Verification items for the finished model (mm, model axes). A direction names the side the tool comes from. Round coordinates to 2 decimals unless told otherwise and drop trailing zeros. Order: outer loops, then holes, each group sorted by start corner. A loop starts at its lowest first (then second) coordinate and runs counter-clockwise, first axis right, second up. Notation, with made-up numbers: (83.5, -8) -> (137.5, -8) arc R25 cw to (137.5, 26) -> close; hole circle Ø8 at (27.25, -36.75). An arc over 180 degrees is marked (long way). Put each result on its own line as item: value.
Autodesk Inventor part; units mm, degrees
ref_plane "YZ Plane" through (0, 0, 0) normal (1, 0, 0) x (0, 1, 0)
ref_plane "XZ Plane" through (0, 0, 0) normal (0, 1, 0) x (-1, 0, 0)
ref_plane "XY Plane" through (0, 0, 0) normal (0, 0, 1) x (1, 0, 0)
sketch "Sketch1" plane through (0, 0, 0) normal (0, 0, 1) x (1, 0, 0)
  point P0 (0, 0)
sketch "Sketch2" plane through (0, 0, 0) normal (0, 0, 1) x (1, 0, 0)
  line L0 (0, 0) -> (215.9, 0)
  line L1 (215.9, 0) -> (215.9, 50.8)
  line L2 (215.9, 50.8) -> (0, 50.8)
  line L3 (0, 50.8) -> (0, 0)
  dimension "d0" = 215.9
  dimension "d1" = 50.8
extrude "Extrusion1" add sketch "Sketch2" along normal blind 9.525
sketch "Sketch3" plane through (0, 0, 9.525) normal (0, 0, 1) x (1, 0, 0)
  line L0 (215.9, 0) -> (215.9, 50.8)
  line L1 (215.9, 0) -> (215.9, 30.48)
  line L2 (0, 0) -> (0, 30.48)
  line L3 (0, 50.8) -> (0, 0)
  line L4 (0, 30.48) -> (215.9, 30.48)
  line L5 (215.9, 0) -> (203.2, 0)
  line L6 (0, 0) -> (215.9, 0)
  line L7 (203.2, 0) -> (203.2, 50.8)
  line L8 (215.9, 50.8) -> (0, 50.8)
  line L9 (203.2, 0) -> (177.8, 0)
  line L10 (177.8, 0) -> (152.4, 0)
  line L11 (177.8, 0) -> (137.16, 0)
  line L12 (177.8, 0) -> (177.8, 9.525)
  line L13 (177.8, 9.525) -> (137.16, 9.525)
  line L14 (137.16, 9.525) -> (177.8, 9.525)
  line L15 (177.8, 9.525) -> (177.8, 30.48)
  line L16 (177.8, 30.48) -> (137.16, 30.48)
  line L17 (137.16, 30.48) -> (137.16, 9.525)
  line L18 (137.16, 9.525) -> (177.36, 9.525)
  line L19 (177.36, 9.525) -> (177.36, 29.525)
  line L20 (177.36, 29.525) -> (137.16, 29.525)
  line L21 (137.16, 29.525) -> (137.16, 9.525)
  point P0 (177.36, 9.525)
  dimension "d4" = 30.48
  dimension "d5" = 30.48
  dimension "d6" = 12.7
  dimension "d7" = 25.4
  dimension "d8" = 25.4
  dimension "d9" = 40.64
  dimension "d10" = 9.525
  dimension "d11" = 40.64
  dimension "d12" = 40.2
  dimension "d13" = 20
extrude "Extrusion2" cut sketch "Sketch3" against normal blind 25.4 contours L13 L17 L20 L19
sketch "Sketch4" plane through (0, 0, 9.525) normal (0, 0, 1) x (1, 0, 0)
  line L0 (0, 0) -> (0, 30.48)
  line L1 (0, 50.8) -> (0, 0)
  line L2 (137.16, 29.525) -> (177.36, 29.525)
  line L3 (0, 30.48) -> (137.16, 29.525)
  line L4 (215.9, 50.8) -> (0, 50.8)
  line L5 (0, 30.48) -> (111.76, 30.48)
  line L6 (111.76, 30.48) -> (111.76, 50.8)
  line L7 (111.76, 50.8) -> (0, 50.8)
  line L8 (0, 50.8) -> (0, 30.48)
  arc A0 (111.76, 40.64) -> (109.4345, 29.525) centre (137.16, 29.525) ccw
  point P0 (109.451, 30.48)
  dimension "d16" = 30.48
extrude "Extrusion3" cut sketch "Sketch4" against normal blind 25.4 contours L4 L6 A0 L5 L1
sketch "Sketch5" plane through (0, 0, 9.525) normal (0, 0, 1) x (1, 0, 0)
  line L0 (137.16, 9.525) -> (177.36, 9.525)
  line L1 (137.16, 9.525) -> (132.36, 9.525)
  line L2 (132.36, 9.525) -> (132.36, 13.9192)
  circle A0 centre (132.36, 13.9192) radius 2.25
  line L3 (132.36, 13.9192) -> (132.36, 23.8192)
  circle A1 centre (132.36, 23.8192) radius 2.2479
  line L4 (177.36, 9.525) -> (182.1606, 9.525)
  line L5 (182.1606, 9.525) -> (182.1606, 13.9192)
  circle A2 centre (182.1606, 13.9192) radius 2.2479
  line L6 (182.1606, 13.9192) -> (182.1606, 23.8252)
  circle A3 centre (182.1606, 23.8252) radius 2.2479
  point P0 (0, 0)
  dimension "d19" = 4.8
  dimension "d20" = 4.3942
  dimension "d21" = 4.5
  dimension "d22" = 9.9
  dimension "d23" = 4.4958
  dimension "d24" = 4.8006
  dimension "d25" = 4.3942
  dimension "d26" = 4.4958
  dimension "d27" = 9.906
  dimension "d28" = 4.4958
extrude "Extrusion4" cut sketch "Sketch5" against normal blind 25.4
sketch "Sketch7" plane through (0, 0, 9.525) normal (0, 0, 1) x (1, 0, 0)
  line L0 (177.36, 29.525) -> (177.36, 9.525)
  line L1 (177.36, 9.525) -> (215.9, 9.525)
  line L2 (215.9, 0) -> (215.9, 50.8)
  circle A0 centre (182.1606, 13.9192) radius 2.2479
  line L3 (184.4085, 13.9192) -> (215.9, 13.9192)
  line L4 (175.586, 50.8) -> (175.586, 0)
  line L5 (0, 0) -> (215.9, 0)
  line L6 (141.0803, 19.525) -> (205.5055, 19.525)
  circle A1 centre (175.586, 19.525) radius 2.2479
  dimension "d33" = 4.4958
extrude "Extrusion6" cut sketch "Sketch7" against normal blind 25.4 contours A1 L6 L0 | L0 L6 L4 A1 | L6 A1 L0 | L0 A1 L4 L6 | L4 L6 A1 | L4 A1 L6
sketch "Sketch8" plane through (0, 0, 9.525) normal (0, 0, 1) x (1, 0, 0)
  point P0 (0, 0)
sketch "Sketch9" plane through (0, 0, 9.525) normal (0, 0, 1) x (1, 0, 0)
  point P0 (0, 0)
sketch "Sketch10" plane through (0, 0, 9.525) normal (0, 0, 1) x (1, 0, 0)
  point P0 (0, 0)
fillet "Fillet1" radius 3.175 4 edges at (137.16, 9.525, 4.7625) (137.16, 29.525, 4.7625) (177.36, 29.525, 4.7625) (177.36, 9.525, 4.7625)
fillet "Fillet2" radius 3.175 3 edges at (111.76, 50.8, 4.7625) (111.76, 40.64, 4.7625) (109.451, 30.48, 4.7625)
fillet "Fillet3" radius 15.24 4 edges at (0, 30.48, 4.7625) (0, 0, 4.7625) (215.9, 50.8, 4.7625) (215.9, 0, 4.7625)
sketch "Sketch11" plane through (0, 0, 9.525) normal (0, 0, 1) x (1, 0, 0)
  line L0 (106.5367, 30.48) -> (15.24, 30.48)
  line L1 (15.24, 0) -> (200.66, 0)
  line L2 (15.24, 30.48) -> (15.24, 0)
  line L3 (15.24, 0) -> (15.24, 15.24)
  line L4 (15.24, 15.24) -> (30.48, 15.24)
  line L5 (30.48, 15.24) -> (0, 15.24)
  arc A0 (15.24, 30.48) -> (15.24, 0) centre (15.24, 15.24) ccw
  circle A1 centre (15.24, 15.24) radius 3.81
  circle A2 centre (25.019, 15.24) radius 1.3589
  circle A3 centre (15.24, 25.019) radius 1.3589
  circle A4 centre (5.461, 15.24) radius 1.3589
  circle A5 centre (15.24, 5.461) radius 1.3589
  point P0 (0, 0)
  dimension "d39" = 15.24
  dimension "d40" = 7.62
  dimension "d41" = 2.7178
  dimension "d42" = 2.7178
  dimension "d43" = 2.7178
  dimension "d44" = 2.7178
extrude "Extrusion7" cut sketch "Sketch11" against normal blind 25.4 contours A2 L4 | L4 A2 | A3 L2 | L2 A3 | A4 L5 | L5 A4 | A1 L4 L2 | L2 L5 A1 | A5 L2 | L2 A5 | L4 A1 L2 | L2 A1 L5
sketch "Sketch12" plane through (0, 0, 9.525) normal (0, 0, 1) x (1, 0, 0)
  circle A0 centre (5.461, 15.24) radius 1.3589
  circle A1 centre (5.461, 15.24) radius 2.2479
  circle A2 centre (15.24, 5.461) radius 1.3589
  circle A3 centre (15.24, 5.461) radius 2.2479
  circle A4 centre (25.019, 15.24) radius 1.3589
  circle A5 centre (25.019, 15.24) radius 2.2479
  circle A6 centre (15.24, 25.019) radius 1.3589
  circle A7 centre (15.24, 25.019) radius 2.2479
  circle A8 centre (15.24, 25.019) radius 2.54
  circle A9 centre (25.019, 15.24) radius 2.54
  circle A10 centre (5.461, 15.24) radius 2.54
  circle A11 centre (15.24, 5.461) radius 2.54
  circle A12 centre (132.36, 13.9192) radius 2.25
  circle A13 centre (132.36, 13.9192) radius 2.54
  circle A14 centre (132.36, 23.8192) radius 2.2479
  circle A15 centre (132.36, 23.8192) radius 2.54
  circle A16 centre (182.1606, 23.8252) radius 2.2479
  circle A17 centre (182.1606, 23.8252) radius 2.54
  circle A18 centre (182.1606, 13.9192) radius 2.2479
  circle A19 centre (182.1606, 13.9192) radius 2.54
  arc A20 (177.36, 18.1445) -> (177.36, 20.9055) centre (175.586, 19.525) ccw
  circle A21 centre (175.586, 19.525) radius 2.54
  point P0 (0, 0)
  dimension "d47" = 4.4958
  dimension "d48" = 4.4958
  dimension "d49" = 4.4958
  dimension "d50" = 4.4958
  dimension "d51" = 5.08
  dimension "d52" = 5.08
  dimension "d53" = 5.08
  dimension "d54" = 5.08
  dimension "d55" = 5.08
  dimension "d56" = 5.08
  dimension "d57" = 5.08
  dimension "d58" = 5.08
  dimension "d59" = 5.08
extrude "Extrusion8" cut sketch "Sketch12" against normal blind 25.4 contours A0 | A1 | A2 | A3 | A4 | A5 | A6 | A7 | A8 | A9 | A10 | A11 | A12 | A13 | A14 | A15 | A16 | A17 | A18 | A19 | A21
sketch "Sketch13" plane through (0, 0, 9.525) normal (0, 0, 1) x (1, 0, 0)
  point P0 (0, 0)
ref_plane "Work Plane1" through (129.9559, 14.7389, 0) normal (1, 0, 0) x (0, 0, -1)
sketch "Sketch14" plane through (129.9559, 14.7389, 0) normal (1, 0, 0) x (0, 0, -1)
  point P0 (0, -14.7389)
sketch "Sketch15" plane through (0, 0, 0) normal (0, 0, -1) x (-1, 0, 0)
  line L0 (-160.2621, 50.5435) -> (-160.2621, 29.525)
  line L1 (-174.185, 29.525) -> (-140.335, 29.525)
  line L2 (-156.9844, 29.525) -> (-156.9844, 39.05)
  line L3 (-109.6833, 39.05) -> (-217.5289, 39.05)
  line L4 (-217.5289, 39.05) -> (-217.5289, 53.1054)
  line L5 (-217.5289, 53.1054) -> (-109.6833, 53.1054)
  line L6 (-109.6833, 53.1054) -> (-109.6833, 39.05)
  point P0 (0, 0)
  point P1 (-184.6931, 29.525)
  point P2 (-129.9559, 29.525)
  dimension "d62" = 9.525
extrude "Extrusion9" cut sketch "Sketch15" against normal blind 25.4 contours L3 L4 L5 L6
fillet "Fillet4" radius 15.24 1 edges at (215.4951, 39.05, 4.7625)
fillet "Fillet5" radius 3.175 1 edges at (111.122, 39.05, 4.7625)
sketch "Sketch16" plane through (0, 0, 9.525) normal (0, 0, 1) x (1, 0, 0)
  line L0 (215.9, 15.24) -> (215.9, 23.81)
  line L1 (215.9, 19.525) -> (178.126, 19.525)
  arc A0 (177.36, 17.7072) -> (177.36, 21.3428) centre (175.586, 19.525) ccw
  arc A1 (200.66, 0) -> (215.9, 15.24) centre (200.66, 15.24) ccw
  line L2 (113.4449, 39.05) -> (200.66, 39.05)
  line L3 (200.66, 0) -> (200.66, 39.05)
  circle A2 centre (200.66, 19.525) radius 2.54
  point P0 (0, 0)
  dimension "d68" = 5.08
extrude "Extrusion10" cut sketch "Sketch16" against normal blind 25.4 contours A2 L3 L1 | L1 L3 A2 | A2 L1 L3 | L1 A2 L3
properties part number "Claw arm"
Item 1: Material ranges on L1, parallel to Y at x = 132.36, z = 3; L2, parallel to Y at x = 15.24, z = 2.75; L3, parallel to Y at x = 158.5, z = 6 (3 decimals), recorded low to high. Write a range as [from, to].
Check sheet entries:
L1: y = [0, 11.38], [16.46, 21.28], [26.36, 39.05]
L2: y = [0, 2.92], [8, 11.43], [19.05, 22.48], [27.56, 30.48]
L3: y = [0, 9.525], [29.525, 39.05]
Item 2: Section check C-C on x = 72. Record the boundary of the cut face in (y, z) (3 decimals).
Check sheet entries:
outline: (0, 0) -> (30.48, 0) -> (30.48, 9.525) -> (0, 9.525) -> close
Item 3: Release check for a two-part mould opening along Y. For faces 1 (the flat face through (60, 30.48, 5)), 2 (the cylindrical face through (16.61, 7.6, 4.83)), 3 (the flat face through (107, 0, 5)) record: +Y half, -Y half, draft (parallel to the pull), parting line (faces both ways), or undercut.
Check sheet entries:
face 1: +Y half
face 2: undercut
face 3: -Y half
Item 4: Section check A-A on x = 166. Record the boundary of the cut face in (y, z) (3 decimals), then the cut area to 3 significant figures.
Check sheet entries:
outline: (0, 0) -> (9.525, 0) -> (9.525, 9.525) -> (0, 9.525) -> close; (29.525, 0) -> (39.05, 0) -> (39.05, 9.525) -> (29.525, 9.525) -> close
area: 181 mm^2
Item 5: Gauge pin test, flat ends, axial feed: pin 1 Ø3 at (x, z) = (184.5, 2) entering from -Y; pin 2 Ø3 at (y, z) = (8.5, 4) entering from -X; pin 3 Ø1 at (y, z) = (5.5, 8) entering from -X; pin 4 Ø1.5 at (y, z) = (14, 5) entering from +X. Record the tip position at first contact, or that the pin passes through.
Check sheet entries:
pin 1: stops at y = 0
pin 2: stops at x = 0.93
pin 3: stops at x = 3.12
pin 4: stops at x = 215.89
Item 6: Section check D-D on z = 4.25. State how many separate pieces and enclosed holes the cut face has, then the cut area to 3 significant figures.
Check sheet entries:
separate pieces: 1
enclosed holes: 11
area: 6,260 mm^2
Item 7: Tool access check on faces 4 (the flat face through (177.36, 15, 5)), 5 (the cylindrical face through (109.98, 35, 4.83)). Record the directions out of +Z, -Z, +X, -X, +Y, -Y that give a thin tool (end or side, any length) a straight path to the whole face; none if there is none.
Check sheet entries:
face 4: +Z, -Z
face 5: +Z, -Z, -X, +Y
Item 8: Section check B-B on x = 132.36. Record the boundary of the cut face in (y, z) (3 decimals).
Check sheet entries:
outline: (0, 0) -> (11.379, 0) -> (11.379, 9.525) -> (0, 9.525) -> close; (16.459, 0) -> (21.279, 0) -> (21.279, 9.525) -> (16.459, 9.525) -> close; (26.359, 0) -> (39.05, 0) -> (39.05, 9.525) -> (26.359, 9.525) -> close
